Input: dimensioned drawing with shaded views. Units: mm. Origin: part minimum x, y, z. Round coordinates to 2 decimals unless told otherwise and drop trailing zeros. Write each loop counter-clockwise with the first axis right and the second up, starting at its lowest first coordinate (ties: lowest second). Pieces come first, ordered by that corner, then holes. Notation, with made-up numbers: M 23.25,62 L 40.25,62 A23 cw 40.25,73 Z; hole C 47.5,83 d9. An arc over 180 degrees is marked long. Put each result on its own line as item: value. Start each with the question number.
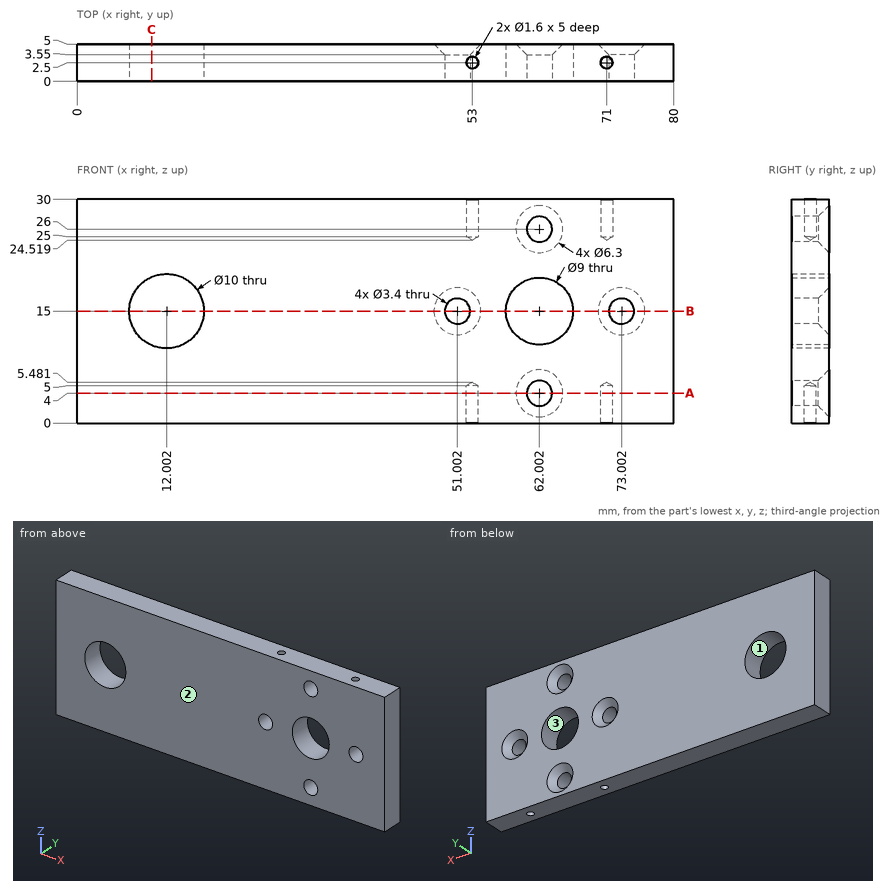
1) Ray query, probe 1 along X at (y, z) = (2.45, 4); probe 2 along Y at (x, z) = (71, 1.4); probe 3 along X at (y, z) = (3.6, 18.25) (1 decimal). Return the intervals inside material, ascending.
2) First-contact query: pin 1 (2.5 mm diameter, centred on x = 71, y = 2.5, fed in from +Z); pin 2 (2 mm diameter, centred on x = 62, z = 26, fed in from -Y) (3 decimals); pin 3 (5.5 mm diameter, centred on x = 73, z = 15, fed in from +Y); pin 4 (1 mm diameter, centred on x = 71, y = 2.5, fed in from -Z). Flat tips, straight axial feed; report the tip coordinate or a pass-through.
3) Section B-B, the plane z = 15. Output: boundary loops of the cut face in (x, y), and give its area (3 significant figures).
4) Section C-C, the plane x = 10. Output: boundary loops of the cut face in (y, z), and give its area (3 significant figures).
5) Draft query along Z for the marked faces 1, 2 and 3. Return one class per face: +Z half, -Z half, draft (parallel to the pull), parting line (faces both ways), or undercut.
6) Section A-A, the plane z = 4. Output: boundary loops of the cut face in (x, y).
Solved:
1. probe 1: x = 0 to 52.2, 53.8 to 60.3, 63.7 to 70.2, 71.8 to 80
1. probe 2: y = 0 to 1.7, 3.3 to 5
1. probe 3: x = 0 to 8.2, 15.8 to 58.9, 65.1 to 80
2. pin 1: stops at z = 30
2. pin 2: passes through
2. pin 3: stops at y = 4.6
2. pin 4: stops at z = 5.18
3. outline: M 0,0 L 7,0 L 7,5 L 0,5 Z; M 17,0 L 49.3,0 L 49.3,3.55 L 47.85,5 L 17,5 Z; M 52.7,0 L 57.5,0 L 57.5,5 L 54.15,5 L 52.7,3.55 Z; M 66.5,0 L 71.3,0 L 71.3,3.55 L 69.85,5 L 66.5,5 Z; M 74.7,0 L 80,0 L 80,5 L 76.15,5 L 74.7,3.55 Z
3. area: 267 mm2
4. outline: M 0,0 L 5,0 L 5,10.42 L 0,10.42 Z; M 0,19.58 L 5,19.58 L 5,30 L 0,30 Z
4. area: 104 mm2
5. face 1: undercut
5. face 2: draft
5. face 3: undercut
6. outline: M 0,0 L 60.3,0 L 60.3,3.55 L 58.85,5 L 0,5 Z; M 63.7,0 L 80,0 L 80,5 L 65.15,5 L 63.7,3.55 Z; hole C 53,2.5 d1.6; hole C 71,2.5 d1.6
